```python
from build123d import *

# Parameters (mm, degrees)
F0_W     = 19
F0_H     = 35
F0_W_2   = 16.2
F0_H_2   = 32.2
F1_DEPTH = 379.987259
F2_R     = 8
F3_DEPTH = 15


with BuildPart() as f1:
    # F0 (on Front) → F1 (new body)
    with BuildSketch(Plane.XZ):
        with Locations((9.5, -17.5)):
            Rectangle(F0_W, F0_H)
        with Locations((9.5, -17.5)):
            Rectangle(F0_W_2, F0_H_2, mode=Mode.SUBTRACT)
    extrude(amount=F1_DEPTH)

    # F2 (on face) → F3 (cut)
    with BuildSketch(Plane.YZ.offset(19)):
        with Locations((-60, -17.5)):
            Circle(F2_R)
    extrude(amount=-F3_DEPTH, mode=Mode.SUBTRACT)


solid = f1.part
```
For this review, take the finished solid that the model builds, in its own axes (mm). A direction names the side the tool comes from. Round coordinates to 2 decimals unless told otherwise and drop trailing zeros. Write each loop counter-clockwise with the first axis right and the second up, starting at its lowest first coordinate (ties: lowest second). Pieces come first, ordered by that corner, then holes. Notation, with made-up numbers: (72.25, 67.5) - (95.25, 67.5) arc R17 ccw to (95.25, 98.5) - close; hole circle Ø8 at (-21, -4). An arc over 180 degrees is marked (long way). Answer as CSV lines item,"result". Start each with the question number.
(1) Machinability: for faces 5 (the flat face through (17.6, -187, -18)), 6 (the flat face through (9, -187, -35)), 7 (the cylindrical face through (18.31, -66.349, -22.368)), which of the approach directions +Z, -Z, +X, -X, +Y, -Y give a long, thin tool a straight path to every point of the face, cutting with its end or side? Answer none if there is none.
(2) Mouldability with a two-part tool opening along X and no side actions: class faces 1 (the flat face through (9, -187, -33.6)), 2 (the flat face through (1, 0, -16)), 3 (the flat face through (1.4, -187, -18)), 4 (the flat face through (19, -187, -18)) as +X half, -X half, draft (parallel to the pull), parting line (faces both ways), or undercut.
(3) Add section A-A, the plane z = -17.5. State the section outline as (x, y) points, plus the area to 3 significant figures.
(4) Add section C-C, the plane y = -160.5. State the section outline as (x, z) points, plus the area to 3 significant figures.
(5) For line 1 (X direction, y = -17, z = -25.5); line 2 (Z direction, x = 18.75, y = -60); line 3 (Z direction, x = 5.75, y = -41.5), list the stretches that pass through material, from the lowest coordinate up.
(6) Add section B-B, the plane x = 6.75. State the section outline as (y, z) points.
(7) Add section D-D, the plane y = -60. State the section outline as (x, z) points.
From the geometry:
1,face 5,"+Y, -Y"
1,face 6,"-Z, +X, -X, +Y, -Y"
1,face 7,"+X"
2,face 1,"undercut"
2,face 2,"draft"
2,face 3,"undercut"
2,face 4,"+X half"
3,outline,"(0, -379.99) - (1.4, -379.99) - (1.4, 0) - (0, 0) - close; (17.6, -379.99) - (19, -379.99) - (19, -68) - (17.6, -68) - close; (17.6, -52) - (19, -52) - (19, 0) - (17.6, 0) - close"
3,area,"1,040 mm²"
4,outline,"(0, -35) - (19, -35) - (19, 0) - (0, 0) - close; hole (1.4, -33.6) - (17.6, -33.6) - (17.6, -1.4) - (1.4, -1.4) - close"
4,area,"143 mm²"
5,line 1,"x = 0 to 1.4, 17.6 to 19"
5,line 2,"z = -35 to -25.5, -9.5 to 0"
5,line 3,"z = -35 to -33.6, -1.4 to 0"
6,outline,"(-379.99, -35) - (0, -35) - (0, -33.6) - (-379.99, -33.6) - close; (-379.99, -1.4) - (0, -1.4) - (0, 0) - (-379.99, 0) - close"
7,outline,"(0, -35) - (19, -35) - (19, -25.5) - (17.6, -25.5) - (17.6, -33.6) - (1.4, -33.6) - (1.4, -1.4) - (17.6, -1.4) - (17.6, -9.5) - (19, -9.5) - (19, 0) - (0, 0) - close"
